Part print with two shaded views. Sizes in mm from the minimum x, y, z corner. A direction names the side the tool comes from. Round coordinates to 2 decimals unless told otherwise and drop trailing zeros. Write each loop counter-clockwise with the first axis right and the second up, starting at its lowest first coordinate (ties: lowest second). Pieces come first, ordered by that corner, then holes. Notation, with made-up numbers: (9.25, 18) -> (31.25, 18) arc R22 cw to (31.25, 49) -> close; hole circle Ø1 at (85, -14). An arc over 180 degrees is marked (long way). Return JSON: item names as keys, results as strings. Group by question number.
(1) Saw through at A-A (y = 3.25). List the corners of the cut face in (x, z).
(2) Saw through at B-B (x = 3.25). List the corners of the cut face in (y, z).
(3) Saw through at C-C (z = 8.25). List the corners of the cut face in (x, y).
(4) Mould opens along X. For the marked faces 1, 2 and 3 say: +X half, -X half, draft (parallel to the pull), parting line (faces both ways), or undercut.
(5) Saw through at D-D (x = 7.25). List the corners of the cut face in (y, z).
(6) Tool access for the marked faces 4, 5 and 6: list every direction of +Z, -Z, +X, -X, +Y, -Y with a clear straight run to the whole face (end or side of a thin tool).
(7) Drill centre lines: L1, parallel to Y at x = 3.25, z = 5.75; L2, parallel to X at y = 3.25, z = 5.5; L3, parallel to Y at x = 3.25, z = 4. Where is each one in solid material? Low to high. Write a range as from..to.
(8) Drop flat-ended pins along their axis: pin 1 Ø3 at (x, y) = (3, 2.5) entering from +Z; pin 2 Ø2 at (y, z) = (3.5, 9.5) entering from -X; pin 3 Ø5 at (x, z) = (14.5, 8) entering from -Y. Give the stop position or say it passes through.
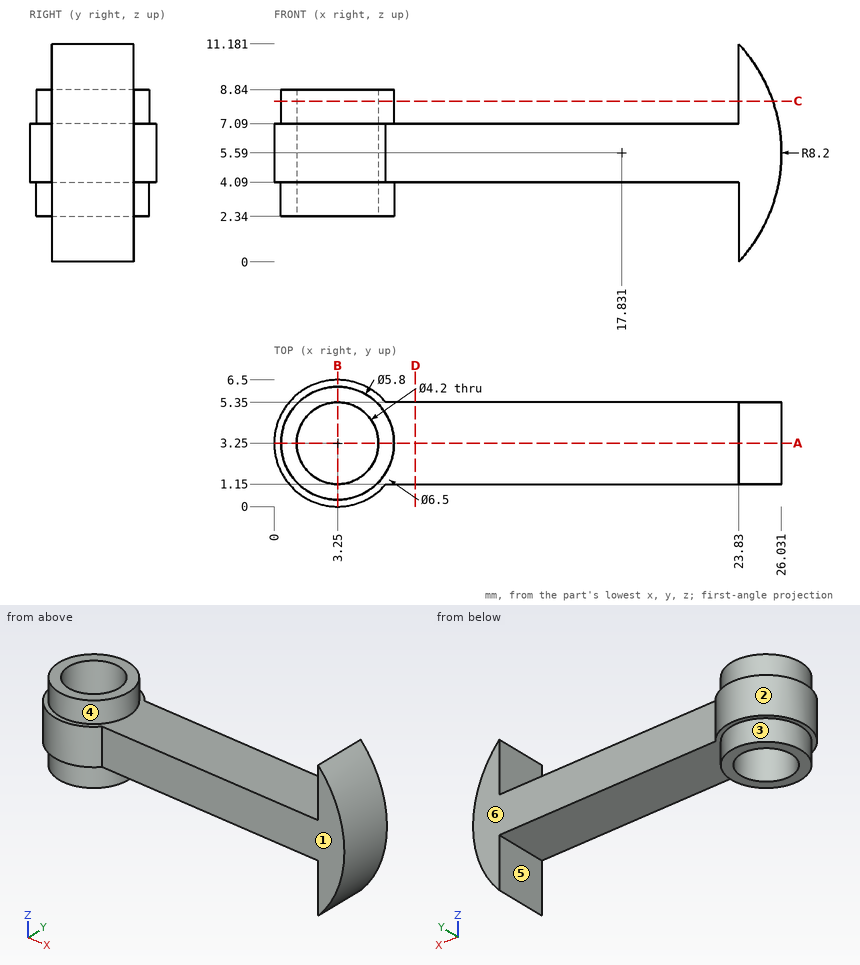
Computed values:
{
 "1": {"outline": "(0, 4.09) -> (0.35, 4.09) -> (0.35, 2.34) -> (1.15, 2.34) -> (1.15, 8.84) -> (0.35, 8.84) -> (0.35, 7.09) -> (0, 7.09) -> close; (5.35, 2.34) -> (6.15, 2.34) -> (6.15, 4.09) -> (23.83, 4.09) -> (23.83, 0) arc R8.2 ccw to (23.83, 11.18) -> (23.83, 7.09) -> (6.15, 7.09) -> (6.15, 8.84) -> (5.35, 8.84) -> close"},
 "2": {"outline": "(0, 4.09) -> (0.35, 4.09) -> (0.35, 2.34) -> (1.15, 2.34) -> (1.15, 8.84) -> (0.35, 8.84) -> (0.35, 7.09) -> (0, 7.09) -> close; (5.35, 2.34) -> (6.15, 2.34) -> (6.15, 4.09) -> (6.5, 4.09) -> (6.5, 7.09) -> (6.15, 7.09) -> (6.15, 8.84) -> (5.35, 8.84) -> close"},
 "3": {"outline": "circle Ø5.8 at (3.25, 3.25); (23.83, 1.15) -> (25.59, 1.15) -> (25.59, 5.35) -> (23.83, 5.35) -> close; hole circle Ø4.2 at (3.25, 3.25)"},
 "4": {"face 1": "draft", "face 2": "parting line", "face 3": "undercut"},
 "5": {"outline": "(1.15, 4.09) -> (5.35, 4.09) -> (5.35, 7.09) -> (1.15, 7.09) -> close"},
 "6": {"face 4": "+Z", "face 5": "-Z, +Y, -Y", "face 6": "+Z, -Z, +X, +Y"},
 "7": {"L1": "0..1.15, 5.35..6.5", "L2": "0..1.15, 5.35..26.03", "L3": "0.35..1.15, 5.35..6.15"},
 "8": {"pin 1": "z = 8.84", "pin 2": "x = 0.35", "pin 3": "y = 1.15"}
}
